Input: part model. Units: mm. Frame: model coordinates. Round coordinates to 2 decimals unless told otherwise and drop trailing zeros. Write each loop counter-clockwise with the first axis right and the second up, starting at its lowest first coordinate (ties: lowest second). Pieces come first, ordered by that corner, then holes. Notation, with made-up numbers: (57.25, 63.25) - (106.25, 63.25) arc R26 cw to (106.25, 96.25) - close; hole circle Ø10 at (27.25, -36.5). An arc over 180 degrees is marked (long way). Use one line per item in the form item = value.
```python
from build123d import *

# Parameters (mm, degrees)
F0_R     = 2
F0_R_2   = 19
F1_DEPTH = 3


with BuildPart() as f1:
    # F0 (on Front) → F1 (new body)
    with BuildSketch(Plane.XZ):
        with BuildLine():
            Line((176.212173, -51.451489), (-185.787827, -51.451489))
            ThreePointArc((-185.787827, -51.451489), (-187.909148, -52.330169), (-188.787827, -54.451489))
            Line((-188.787827, -54.451489), (-188.787827, -114.451489))
            Line((-188.787827, -114.451489), (179.212173, -114.451489))
            Line((179.212173, -114.451489), (179.212173, -54.451489))
            ThreePointArc((179.212173, -54.451489), (178.333493, -52.330169), (176.212173, -51.451489))
        make_face()
        with Locations((-167.960797, -100.951489)):
            Circle(F0_R, mode=Mode.SUBTRACT)
        with Locations((-134.960797, -100.951489)):
            Circle(F0_R, mode=Mode.SUBTRACT)
        with Locations((-151.460797, -84.451489)):
            Circle(F0_R_2, mode=Mode.SUBTRACT)
        with Locations((-167.960797, -67.951489)):
            Circle(F0_R, mode=Mode.SUBTRACT)
        with Locations((-134.960797, -67.951489)):
            Circle(F0_R, mode=Mode.SUBTRACT)
    extrude(amount=F1_DEPTH)


solid = f1.part
```
(1) First-contact query: pin 1 Ø5 at (x, z) = (-99.5, -86) entering from +Y. Flat tip, straight axial feed; report the tip coordinate or a pass-through.
Derived:
pin_1 = 0
(2) Cut plane B-B on x = -148.5. Output: boundary loops of the cut face in (y, z).
Derived:
outline = (-3, -114.45) - (0, -114.45) - (0, -103.22) - (-3, -103.22) - close; (-3, -65.68) - (0, -65.68) - (0, -51.45) - (-3, -51.45) - close
(3) Cut plane A-A on z = -79. Output: boundary loops of the cut face in (x, y), then the cut area to 3 significant figures.
Derived:
outline = (-188.79, -3) - (-169.66, -3) - (-169.66, 0) - (-188.79, 0) - close; (-133.26, -3) - (179.21, -3) - (179.21, 0) - (-133.26, 0) - close
area = 995 mm^2
(4) Material intervals for L1, parallel to X at y = -1.9, z = -83; L2, parallel to Z at x = -156, y = -2; L3, parallel to X at y = -2.2, z = -85, sorted ascending.
Derived:
L1 = -188.79 to -170.41, -132.52 to 179.21
L2 = -114.45 to -102.9, -66 to -51.45
L3 = -188.79 to -170.45, -132.47 to 179.21
(5) Cut plane C-C on y = -2.4. Output: boundary loops of the cut face in (x, z), then the cut area to 3 significant figures.
Derived:
outline = (-188.79, -114.45) - (179.21, -114.45) - (179.21, -54.45) arc R3 ccw to (176.21, -51.45) - (-185.79, -51.45) arc R3 ccw to (-188.79, -54.45) - close; hole circle Ø38 at (-151.46, -84.45); hole circle Ø4 at (-167.96, -100.95); hole circle Ø4 at (-167.96, -67.95); hole circle Ø4 at (-134.96, -100.95); hole circle Ø4 at (-134.96, -67.95)
area = 22,000 mm^2
(6) Draft query along X for faces 1 (the face through (-133.34, -1.48, -78.74)), 2 (the face through (-7, -3, -83)). Return one class per face: released by +X, released by -X, zero draft, split by the parting line, or undercut.
Derived:
face_1 = undercut
face_2 = zero draft
